```python
from build123d import *

# Parameters (mm, degrees)
SKETCH_1_W          = 20
SKETCH_1_H          = 15
EXTRUDE_1_DEPTH     = 16
FILLET_1_R          = 3.5
SKETCH_2_W          = 13
SKETCH_2_H          = 9
EXTRUDE_2_DEPTH     = 4
FILLET_2_R          = 0.5
EXTRUDE_3_DEPTH     = 10
SKETCH_4_W          = 9
SKETCH_4_H          = 10
CUT_EXTRUDE_2_DEPTH = 0.7
SKETCH_5_R          = 4.120834068
CUT_EXTRUDE_3_DEPTH = 1
CUT_EXTRUDE_5_DEPTH = 13
SKETCH_7_W          = 9
SKETCH_7_H          = 1.011185769
EXTRUDE_4_DEPTH     = 9
FILLET_3_R          = 0.5
CUT_EXTRUDE_6_DEPTH = 9


with BuildPart() as part:
    # ｽｹｯﾁ1 → ﾎﾞｽ - 押し出し1 (new body)
    with BuildSketch(Plane.XY):
        with Locations((10, 7.5)):
            Rectangle(SKETCH_1_W, SKETCH_1_H)
    extrude(amount=EXTRUDE_1_DEPTH)

    # ﾌｨﾚｯﾄ1
    fillet_1_edges = [part.edges().sort_by_distance(p)[0] for p in [
        (20, 7.5, 16),
        (0, 7.5, 16),
        (20, 7.5, 0),
        (0, 7.5, 0),
    ]]
    fillet(fillet_1_edges, radius=FILLET_1_R)

    # ｽｹｯﾁ2 → ﾎﾞｽ - 押し出し2 (add)
    with BuildSketch(Plane(origin=(0, 0, 0), x_dir=(-1, 0, 0), z_dir=(0, 0, -1))):
        with Locations((-10, 10.5)):
            Rectangle(SKETCH_2_W, SKETCH_2_H)
    extrude(amount=EXTRUDE_2_DEPTH)

    # ﾌｨﾚｯﾄ2
    fillet_2_edges = [part.edges().sort_by_distance(p)[0] for p in [
        (16.5, 10.5, -4),
        (10, 6, -4),
        (3.5, 10.5, -4),
    ]]
    fillet(fillet_2_edges, radius=FILLET_2_R)

    # ｽｹｯﾁ3 → ﾎﾞｽ - 押し出し3 (add)
    with BuildSketch(Plane.XZ):
        with BuildLine():
            Line((3.5, 16), (5.627627053, 13.041328389))
            ThreePointArc((5.627627053, 13.041328389), (4.172978297, 10.083248698), (5.821248207, 7.228525459))
            Line((5.821248207, 7.228525459), (3.5, 3.5))
            Line((3.5, 3.5), (3.5, 0))
            Line((3.5, 0), (16.5, 0))
            Line((16.5, 0), (16.5, 3.5))
            Line((16.5, 3.5), (14.565352324, 6.9904115))
            ThreePointArc((14.565352324, 6.9904115), (16.668731913, 10.163952157), (14.630738056, 13.379873028))
            Line((14.630738056, 13.379873028), (16.5, 16))
            Line((16.5, 16), (3.5, 16))
        make_face()
    extrude(amount=EXTRUDE_3_DEPTH)

    # ｽｹｯﾁ4 → ｶｯﾄ - 押し出し2 (cut)
    with BuildSketch(Plane.XY.offset(16)):
        with Locations((10, -5)):
            Rectangle(SKETCH_4_W, SKETCH_4_H)
    extrude(amount=-CUT_EXTRUDE_2_DEPTH, mode=Mode.SUBTRACT)

    # ｽｹｯﾁ5 → ｶｯﾄ - 押し出し3 (cut)
    with BuildSketch(Plane.XZ.offset(10)):
        with Locations(Location((10, 10.403392153, 0), (0, 0, 270))):
            Circle(SKETCH_5_R)
    extrude(amount=-CUT_EXTRUDE_3_DEPTH, mode=Mode.SUBTRACT)

    # ｽｹｯﾁ6 → ｶｯﾄ - 押し出し5 (cut)
    with BuildSketch(Plane(origin=(0, 15, 0), x_dir=(1, 0, 0), z_dir=(0, 1, 0))):
        with BuildLine():
            Line((15.5, 3), (4.5, 3))
            Line((4.5, 3), (4.5, -1.208712153))
            ThreePointArc((4.5, -1.208712153), (2.130693606, -1.408349934), (1, -3.5))
            Line((1, -3.5), (1, -12.5))
            ThreePointArc((1, -12.5), (1.732233047, -14.267766953), (3.5, -15))
            Line((3.5, -15), (16.5, -15))
            ThreePointArc((16.5, -15), (18.267766953, -14.267766953), (19, -12.5))
            Line((19, -12.5), (19, -3.5))
            ThreePointArc((19, -3.5), (17.869306394, -1.408349934), (15.5, -1.208712153))
            Line((15.5, -1.208712153), (15.5, 3))
        make_face()
    extrude(amount=-CUT_EXTRUDE_5_DEPTH, mode=Mode.SUBTRACT)

    # ｽｹｯﾁ7 → ﾎﾞｽ - 押し出し4 (add)
    with BuildSketch(Plane(origin=(0, 2, 0), x_dir=(1, 0, 0), z_dir=(0, 1, 0))):
        with Locations((10, -0.505592885)):
            Rectangle(SKETCH_7_W, SKETCH_7_H)
    extrude(amount=EXTRUDE_4_DEPTH)

    # ﾌｨﾚｯﾄ3
    fillet_3_edges = [part.edges().sort_by_distance(p)[0] for p in [
        (5.5, 11, 0.505592885),
        (10, 11, 1.011185769),
        (14.5, 11, 0.505592885),
        (10, 11, 0),
    ]]
    fillet(fillet_3_edges, radius=FILLET_3_R)

    # ｽｹｯﾁ8 → ｶｯﾄ - 押し出し6 (cut)
    with BuildSketch(Plane.XZ.offset(10)):
        with BuildLine():
            Line((4.5, 1), (4.5, 0))
            Line((4.5, 0), (5.838412619, 0))
            Line((5.838412619, 0), (5.838412619, 1))
            Line((5.838412619, 1), (14.187040515, 1))
            Line((14.187040515, 1), (14.187040515, 0))
            Line((14.187040515, 0), (15.5, 0))
            Line((15.5, 0), (15.5, 1))
            Line((15.5, 1), (15.5, 3.241396329))
            Line((15.5, 3.241396329), (13.566856979, 6.729093192))
            ThreePointArc((13.566856979, 6.729093192), (10.11032626, 5.283746689), (6.594740038, 6.578846932))
            Line((6.594740038, 6.578846932), (4.5, 3.214152221))
            Line((4.5, 3.214152221), (4.5, 1))
        make_face()
    extrude(amount=-CUT_EXTRUDE_6_DEPTH, mode=Mode.SUBTRACT)


solid = part.part
```
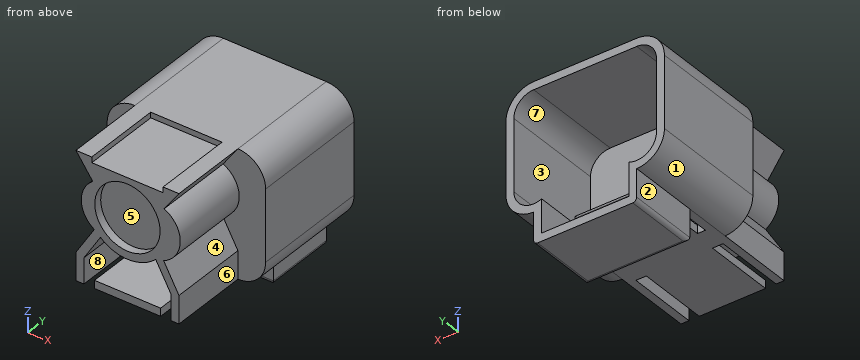
Source: CAD feature listing. Evaluate the final solid. Frame: model axes, mm. Face numbers are marked on the shaded views. A direction names the side the tool comes from. Give positions to 0.01 mm unless a question says otherwise; leave off trailing zeros. Loops run counter-clockwise (first coordinate to the right, second up) from the corner with the lowest first, then second, coordinate; pieces in that order, holes last. Notation, with made-up numbers: (24.25, -34.75) - (82.25, -34.75) arc R25 ccw to (82.25, -3.75) - close; hole circle Ø9 at (-37.5, -39.75). An arc over 180 degrees is marked (long way). Use CSV: the item, a comma, the result in double quotes. Start each with the question number.
1. Section D-D (y = 5). Output: boundary loops of the cut face in (x, z), then the cut area to 3 significant figures.
2. Draft query along Z for the marked faces 1, 2 and 3. Return one class per face: +Z half, -Z half, draft (parallel to the pull), parting line (faces both ways), or undercut.
3. Pin query (flat end, axial travel): pin 1 (1.8 mm diameter, centred on y = 10, z = -1.5, fed in from +X); pin 2 (8 mm diameter, centred on y = -7, z = 5.5, fed in from -X); pin 3 (2.5 mm diameter, centred on x = 10, z = 8.5, fed in from -Y). Return the tip coordinate at first contact, or that it passes through.
4. Section B-B (y = -3.25). Output: boundary loops of the cut face in (x, z), then the cut area to 3 significant figures.
5. Reachability of the marked faces 4, 5, 6, 7 and 8 from +Z, -Z, +X, -X, +Y, -Y: full face, straight path, thin tool, end or side. Return the list, or none.
6. Section A-A (y = 8.75). Output: boundary loops of the cut face in (x, z).
7. Ray query, L1, parallel to X at y = -7.25, z = 0.5; L2, parallel to X at y = -5.75, z = 1.5; L3, parallel to X at y = 10.75, z = 11.5. Return the intervals inside material, ascending.
Response:
1,outline,"(0, 3.5) arc R3.5 ccw to (3.5, 0) - (4.5, 0) - (4.5, 1.21) arc R2.5 cw to (1, 3.5) - (1, 12.5) arc R2.5 cw to (3.5, 15) - (16.5, 15) arc R2.5 cw to (19, 12.5) - (19, 3.5) arc R2.5 cw to (15.5, 1.21) - (15.5, 0) - (16.5, 0) arc R3.5 ccw to (20, 3.5) - (20, 12.5) arc R3.5 ccw to (16.5, 16) - (3.5, 16) arc R3.5 ccw to (0, 12.5) - close; (5.5, 0) - (14.5, 0) - (14.5, 1.01) - (5.5, 1.01) - close"
1,area,"61.1 mm²"
2,face 1,"-Z half"
2,face 2,"draft"
2,face 3,"undercut"
3,pin 1,"x = 16.5"
3,pin 2,"x = 3.5"
3,pin 3,"y = -9"
4,outline,"(3.5, 0) - (4.5, 0) - (4.5, 3.21) - (6.59, 6.58) arc R5.12 ccw to (13.57, 6.73) - (15.5, 3.24) - (15.5, 0) - (16.5, 0) - (16.5, 3.5) - (14.57, 6.99) arc R3.5 ccw to (14.63, 13.38) - (16.5, 16) - (14.5, 16) - (14.5, 15.3) - (5.5, 15.3) - (5.5, 16) - (3.5, 16) - (5.63, 13.04) arc R3.5 ccw to (5.82, 7.23) - (3.5, 3.5) - close; (5.84, 0) - (14.19, 0) - (14.19, 1) - (5.84, 1) - close"
4,area,"128 mm²"
5,face 4,"+X, -Y"
5,face 5,"-Y"
5,face 6,"-Z, +X, -Y"
5,face 7,"+Y"
5,face 8,"-Z, -Y"
6,outline,"(0, 3.5) arc R3.5 ccw to (3.5, 0) - (3.5, -3.5) arc R0.5 ccw to (4, -4) - (16, -4) arc R0.5 ccw to (16.5, -3.5) - (16.5, 0) arc R3.5 ccw to (20, 3.5) - (20, 12.5) arc R3.5 ccw to (16.5, 16) - (3.5, 16) arc R3.5 ccw to (0, 12.5) - close; (5.5, 0) - (14.5, 0) - (14.5, 1.01) - (5.5, 1.01) - close; hole (1, 3.5) arc R2.5 ccw to (4.5, 1.21) - (4.5, -3) - (15.5, -3) - (15.5, 1.21) arc R2.5 ccw to (19, 3.5) - (19, 12.5) arc R2.5 ccw to (16.5, 15) - (3.5, 15) arc R2.5 ccw to (1, 12.5) - close"
7,L1,"3.5 to 4.5, 5.84 to 14.19, 15.5 to 16.5"
7,L2,"3.5 to 4.5, 15.5 to 16.5"
7,L3,"0 to 1, 19 to 20"
